Part model, mm, in its own coordinate system. A direction names the side the tool comes from. Coordinates: 2 decimals unless noted, no trailing zeros. Loops run counter-clockwise (first coordinate to the right, second up) from the corner with the lowest first, then second, coordinate; pieces in that order, holes last. Notation, with made-up numbers: (-10.75, 25) -> (17.25, 25) arc R22 ccw to (17.25, 45) -> close; hole circle Ø7 at (43.25, -17.5). An arc over 180 degrees is marked (long way). One line per question, with ' | ' between items. Start each with the question number.
1) Cut at D-D (x = 12.5). List the corners of the cut face in (y, z), plus the area to 3 significant figures.
2) Drop flat-ended pins along their axis: pin 1 (2 mm diameter, centred on y = -11, z = 0, fed in from -X); pin 2 (11 mm diameter, centred on x = 0, y = 0, fed in from -Z); pin 3 (5 mm diameter, centred on x = 0, y = 0, fed in from -Z); pin 4 (1 mm diameter, centred on x = 12, y = 5.5, fed in from +Z). Give the stop position or say it passes through.
3) Two-plate mould, pull along Y, no slides. Class faces 3 (the face through (-4.434, 3.4, 0.273)), 4 (the face through (2, -4, 3.492)), 5 (the face through (1.885, 14.355, -3.814)), 6 (the face through (0, -6, -2.858)): released by +Y, released by -Y, zero draft, split by the parting line, or undercut.
4) Probe L1, parallel to Y at x = 0, z = 1.5; L2, parallel to Y at x = -2.5, z = -0.5; L3, parallel to X at y = -3.5, z = -2.5. List the from-to ranges inside material, lowest first. Write a range as from..to.
5) Cut at A-A (x = 0). List the corners of the cut face in (y, z), plus the area to 3 significant figures.
6) Cut at C-C (y = 5). List the corners of the cut face in (x, z), plus the area to 3 significant figures.
7) Cut at B-B (z = -1). List the corners of the cut face in (x, y), plus the area to 3 significant figures.
8) 3-axis set-ups, long thin cutter, end or side, ignore diameter. For faces 1 (the face through (7, -13, -3.492)), 2 (the face through (3.4, -3, -4.128)): which of +Z, -Z, +X, -X, +Y, -Y reach the whole face in a straight line?
Autodesk Inventor part; units mm, degrees
ref_plane "YZ Plane" through (0, 0, 0) normal (1, 0, 0) x (0, 1, 0)
ref_plane "XZ Plane" through (0, 0, 0) normal (0, 1, 0) x (-1, 0, 0)
ref_plane "XY Plane" through (0, 0, 0) normal (0, 0, 1) x (1, 0, 0)
sketch "Sketch1" plane through (0, 0, 0) normal (0, 0, 1) x (1, 0, 0)
  circle A0 centre (0, 0) radius 5.588
  circle A1 centre (0, 0) radius 4.318
  circle A2 centre (0, 0) radius 14.478
  circle A3 centre (0, 0) radius 15.748
  dimension "d1" = 11.176
  dimension "d2" = 1.27
  dimension "d3" = 8.89
  dimension "d4" = 1.27
extrude "Extrusion1" add sketch "Sketch1" along normal mid plane 6.985
sketch "Sketch5" plane through (0, 0, -3.4925) normal (0, 0, -1) x (-1, 0, 0)
  circle A0 centre (0, 0) radius 14.478
  circle A1 centre (0, 0) radius 15.748
  circle A2 centre (0, 0) radius 4.318
  circle A3 centre (0, 0) radius 5.588
extrude "Extrusion3" add sketch "Sketch5" along normal mid plane 1.27 contours A0 | A3
sketch "Sketch6" plane through (0, 0, -4.1275) normal (0, 0, -1) x (-1, 0, 0)
  circle A0 centre (0, 0) radius 14.478
  arc A1 (-3.1559, 14.1299) -> (3.1559, 14.1299) centre (0, 14.478) ccw
  dimension "d17" = 6.35
properties part number "Wheel"
Reported:
1) outline: (-9.58, -3.49) -> (-7.3, -3.49) -> (-7.3, -4.13) -> (7.3, -4.13) -> (7.3, -3.49) -> (9.58, -3.49) -> (9.58, 3.49) -> (7.3, 3.49) -> (7.3, -2.86) -> (-7.3, -2.86) -> (-7.3, 3.49) -> (-9.58, 3.49) -> close | area: 50.3 mm²
2) pin 1: stops at x = -12.17 | pin 2: stops at z = -4.13 | pin 3: passes through | pin 4: stops at z = -2.86
3) face 3: undercut | face 4: zero draft | face 5: split by the parting line | face 6: undercut
4) L1: y = -15.75..-14.48, -5.59..-4.32, 4.32..5.59, 14.48..15.75 | L2: y = -15.55..-14.26, -5..-3.52, 3.52..5, 14.26..15.55 | L3: x = -15.35..-14.05, -4.36..-2.53, 2.53..4.36, 14.05..15.35
5) outline: (-15.75, -3.49) -> (-14.48, -3.49) -> (-14.48, -4.13) -> (-4.32, -4.13) -> (-4.32, 3.49) -> (-5.59, 3.49) -> (-5.59, -2.86) -> (-14.48, -2.86) -> (-14.48, 3.49) -> (-15.75, 3.49) -> close; (4.32, -4.13) -> (14.48, -4.13) -> (14.48, -3.49) -> (15.75, -3.49) -> (15.75, 3.49) -> (14.48, 3.49) -> (14.48, -2.86) -> (5.59, -2.86) -> (5.59, 3.49) -> (4.32, 3.49) -> close | area: 59.7 mm²
6) outline: (-14.93, -3.49) -> (-13.59, -3.49) -> (-13.59, -4.13) -> (13.59, -4.13) -> (13.59, -3.49) -> (14.93, -3.49) -> (14.93, 3.49) -> (13.59, 3.49) -> (13.59, -2.86) -> (2.5, -2.86) -> (2.5, 3.49) -> (-2.5, 3.49) -> (-2.5, -2.86) -> (-13.59, -2.86) -> (-13.59, 3.49) -> (-14.93, 3.49) -> close | area: 85.0 mm²
7) outline: circle Ø31.5 at (0, 0); circle Ø11.18 at (0, 0); hole circle Ø28.96 at (0, 0); hole circle Ø8.64 at (0, 0) | area: 160 mm²
8) face 1: -Z | face 2: -Z, +X, -X, +Y, -Y
